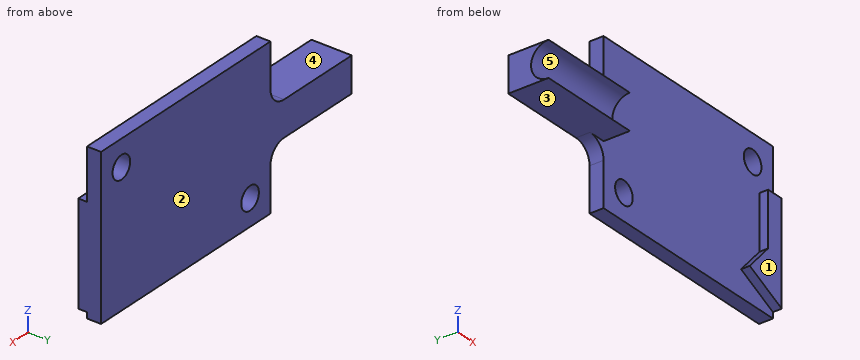
from build123d import *

# Parameters (mm, degrees)
BOSS_EXTRUDE1_DEPTH = 1.6
BOSS_EXTRUDE2_DEPTH = 12
SKETCH3_R           = 1.3
CUT_EXTRUDE1_DEPTH  = 1.6
FILLET1_R           = 2
BOSS_EXTRUDE3_DEPTH = 1


with BuildPart() as part:
    # Sketch1 → Boss-Extrude1 (new body)
    with BuildSketch(Plane(origin=(0, 0, 0), x_dir=(1, 0, 0), z_dir=(0, 1, 0))):
        Polygon((0, 11), (0, 18), (25, 18), (25, 0), (0, 0), (0, 7), (-12, 7), (-12, 11), align=None)
    extrude(amount=BOSS_EXTRUDE1_DEPTH)

    # Sketch2 → Boss-Extrude2 (add)
    with BuildSketch(Plane.ZY.offset(12)):
        with BuildLine():
            Line((-7, -3), (-7, 0))
            Line((-7, 0), (-11, 0))
            Line((-11, 0), (-11, -3))
            ThreePointArc((-11, -3), (-9, -1), (-7, -3))
        make_face()
    extrude(amount=-BOSS_EXTRUDE2_DEPTH)

    # Sketch3 → Cut-Extrude1 (cut)
    with BuildSketch(Plane(origin=(0, 1.6, 0), x_dir=(1, 0, 0), z_dir=(0, 1, 0))):
        with Locations((3, 15)):
            Circle(SKETCH3_R)
        with Locations((22, 3)):
            Circle(SKETCH3_R)
    extrude(amount=-CUT_EXTRUDE1_DEPTH, mode=Mode.SUBTRACT)

    # Fillet1
    fillet1_edges = [part.edges().sort_by_distance(p)[0] for p in [
        (0, 0.8, -7),
        (0, 0.8, -11),
    ]]
    fillet(fillet1_edges, radius=FILLET1_R)

    # Sketch4 → Boss-Extrude3 (add)
    with BuildSketch(Plane.XZ):
        Polygon((25, -5.8), (25, -17.33), (20.285605544, -15.019808468), (23, -11.947014506), (23, -5.8), align=None)
    extrude(amount=BOSS_EXTRUDE3_DEPTH)


solid = part.part
Model file for the job. Use its own axes, mm. Face numbers are marked on the shaded views. A direction names the side the tool comes from. Give positions to 0.01 mm unless a question says otherwise; leave off trailing zeros. Order: outer loops, then holes, each group sorted by start corner. A loop starts at its lowest first (then second) coordinate and runs counter-clockwise, first axis right, second up. Notation, with made-up numbers: (3.25, 88) - (43.25, 88) arc R18 ccw to (43.25, 115) - close; hole circle Ø2 at (31, 58). An arc over 180 degrees is marked (long way). Return JSON: item names as keys, results as strings.
1) Probe line 1 (X direction, y = 0.5, z = -3); line 2 (X direction, y = 0.9, z = -15); line 3 (Y direction, x = 12, z = -13). List the from-to ranges inside material, lowest first. Write a range as from..to.
Geometry says:
{"line 1": "0..20.7, 23.3..25", "line 2": "0..1.7, 4.3..25", "line 3": "0..1.6"}
2) 3-axis set-ups, long thin cutter, end or side, ignore diameter. For the marked faces 1 and 2: which of +Z, -Z, +X, -X, +Y, -Y reach the whole face in a straight line?
Geometry says:
{"face 1": "+Z, -Z, +X, -Y", "face 2": "+Z, -Z, +X, -X, +Y"}
3) Cut at D-D, the plane z = -9. Give the cut face in (x, y), plus the area to 3 significant figures.
Geometry says:
{"outline": "(-12, -1) - (0, -1) - (0, 0) - (23, 0) - (23, -1) - (25, -1) - (25, 1.6) - (-12, 1.6) - close", "area": "73.2 mm²"}
4) Pull direction Z, two halves, no side cores. Call the marked faces 3, 4 and 5: pulls with the +Z half, pulls with the -Z half, needs draft (parallel to the pull), parting line crosses it, or undercut.
Geometry says:
{"face 3": "pulls with the -Z half", "face 4": "pulls with the +Z half", "face 5": "undercut"}
5) Cut at B-B, the plane z = -3. Give the cut face in (x, y), plus the area to 3 significant figures.
Geometry says:
{"outline": "(0, 0) - (20.7, 0) - (20.7, 1.6) - (0, 1.6) - close; (23.3, 0) - (25, 0) - (25, 1.6) - (23.3, 1.6) - close", "area": "35.8 mm²"}
6) Cut at A-A, the plane y = 0.5. Give the cut face in (x, z), plus the area to 3 significant figures.
Geometry says:
{"outline": "(-12, -11) - (-2, -11) arc R2 cw to (0, -13) - (0, -18) - (25, -18) - (25, 0) - (0, 0) - (0, -5) arc R2 cw to (-2, -7) - (-12, -7) - close; hole circle Ø2.6 at (3, -15); hole circle Ø2.6 at (22, -3)", "area": "489 mm²"}
7) Flat gauge pins, fed straight in: P1, Ø1.4, axis at x = -3.5, y = -1, coming from the -Z side; P2, Ø4, axis at x = 22, z = -12, coming from the -Y side; P3, Ø8, axis at x = 12.5, z = -15, coming from the -Y side. Where does each tip first touch, or does it go through?
Geometry says:
{"P1": "z = -11", "P2": "y = -1", "P3": "y = 0"}
